Model file for the job. Use its own axes, mm. Face numbers are marked on the shaded views. A direction names the side the tool comes from. Coordinates: 2 decimals unless noted, no trailing zeros. Write each loop counter-clockwise with the first axis right and the second up, starting at its lowest first coordinate (ties: lowest second). Pieces come first, ordered by that corner, then holes.
Q1. Drill centre lines: probe 1 along X at (y, z) = (12.25, 13); probe 2 along Y at (x, z) = (9.75, 16.75); probe 3 along Z at (x, y) = (12.5, 19.5). Where is each one in solid material? Low to high.
Q2. Which spindle directions (+Z, -Z, +X, -X, +Y, -Y) get a long thin tool onto all of the face, cutting with end or side? Do the marked faces 5, 6, 7, 8 and 9. Say none if no direction does.
Q3. Band-saw the part on C-C, the plane z = 17.5. Write the cut outline in (x, y).
Q4. Pull direction Y, two halves, no side cores. Call the marked faces 1, 2, 3 and 4: released by +Y, released by -Y, zero draft, split by the parting line, or undercut.
Q5. Band-saw the part on B-B, the plane y = 10.5. Write the cut outline in (x, z) (3 decimals), plus the area to 3 significant figures.
Q6. Band-saw the part on D-D, the plane y = 2.5. Write the cut outline in (x, z), plus the area to 3 significant figures.
Q7. Band-saw the part on A-A, the plane x = 8.25. Write the cut outline in (y, z).
Q8. Pin check, flat tips, straight feed: P1, Ø3.5, axis at x = 9, y = 16.5, coming from the -Z side; P2, Ø3.5, axis at x = 7.5, z = 8.5, coming from the +Y side. Stop position of each tip, or through.
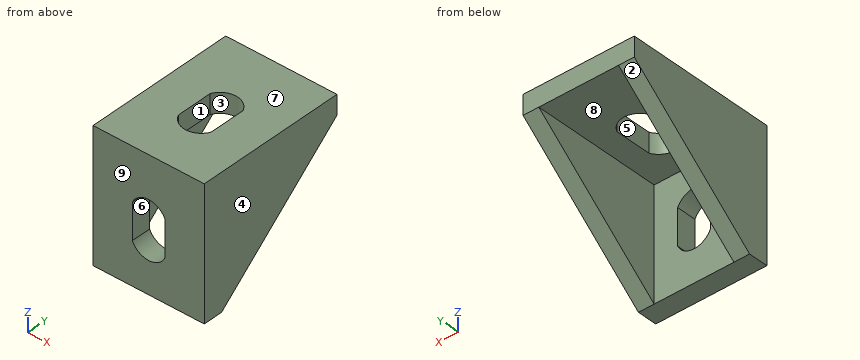
Autodesk Inventor part; units mm, degrees
ref_plane "YZ Plane" through (0, 0, 0) normal (1, 0, 0) x (0, 1, 0)
ref_plane "XZ Plane" through (0, 0, 0) normal (0, 1, 0) x (-1, 0, 0)
ref_plane "XY Plane" through (0, 0, 0) normal (0, 0, 1) x (1, 0, 0)
sketch "Sketch1" plane through (0, 0, 0) normal (0, 0, 1) x (1, 0, 0)
  line L0 (0, 0) -> (0, 3)
  line L1 (0, 3) -> (17, 3)
  line L2 (17, 3) -> (17, 0)
  line L3 (17, 0) -> (0, 0)
  dimension "d0" = 3
  dimension "d1" = 17
extrude "Extrusion1" add sketch "Sketch1" along normal blind 20
sketch "Sketch2" plane through (17, 0, 0) normal (1, 0, 0) x (0, 0, -1)
  point P0 (0, 0)
sketch "Sketch3" plane through (0, 3, 0) normal (0, 1, 0) x (1, 0, 0)
  line L0 (17, -20) -> (17, -17)
  line L1 (17, 0) -> (17, -20)
  line L2 (17, -17) -> (0, -17)
  line L3 (0, 0) -> (0, -20)
  line L4 (17, -20) -> (0, -20)
  line L5 (0, -20) -> (0, -17)
  line L6 (0, -20) -> (17, -20)
  dimension "d4" = 3
extrude "Extrusion2" add sketch "Sketch3" along normal blind 20
sketch "Sketch4" plane through (17, 0, 0) normal (1, 0, 0) x (0, 0, -1)
  line L0 (-20, 23) -> (-17, 23)
  line L1 (0, 3) -> (-17, 23)
  line L2 (0, 3) -> (-17, 3)
  line L3 (-17, 23) -> (-17, 3)
  line L4 (-17, 3) -> (0, 3)
  point P0 (0, 0)
extrude "Extrusion3" add sketch "Sketch4" against normal blind 2.4
sketch "Sketch5" plane through (0, 0, 0) normal (-1, 0, 0) x (0, 0, 1)
  line L0 (17, 3) -> (17, 23)
  line L1 (0, 3) -> (0, 0)
  line L2 (17, 23) -> (0, 3)
  line L3 (0, 3) -> (17, 3)
  line L4 (17, 23) -> (0, 3)
  line L5 (17, 3) -> (17, 23)
extrude "Extrusion4" add sketch "Sketch5" against normal blind 2.4
sketch "Sketch6" plane through (14.6, 3, 17) normal (0, 0, -1) x (-1, 0, 0)
  line L0 (-2.4, -3) -> (-2.4, 20)
  line L1 (-2.4, -3) -> (6.1, -3)
  line L2 (14.6, -3) -> (-2.4, -3)
  line L3 (6.1, 5) -> (6.7519, 5)
  line L4 (6.7519, 10.5) -> (6.1, 10.5)
  line L5 (6.1, 10.5) -> (3.6, 10.5)
  line L6 (3.6, 10.5) -> (8.6, 10.5)
  line L7 (6.1, 5) -> (3.6, 5)
  line L8 (3.6, 5) -> (8.6, 5)
  line L9 (8.6, 5) -> (8.6, 10.5)
  line L10 (3.6, 10.5) -> (3.6, 5)
  arc A0 (8.6, 10.5) -> (3.6, 10.5) centre (6.1, 9.3544) ccw
  arc A1 (3.6, 5) -> (8.6, 5) centre (6.1, 6.1456) ccw
  dimension "d11" = 8.5
extrude "Extrusion5" cut sketch "Sketch6" against normal through all
sketch "Sketch7" plane through (2.4, 3, 17) normal (0, 1, 0) x (1, 0, 0)
  line L0 (-2.4, -3) -> (-2.4, 20)
  line L1 (-2.4, -3) -> (6.1, -3)
  line L2 (14.6, -3) -> (-2.4, -3)
  line L3 (6.1, 5) -> (6.7519, 5)
  line L4 (6.7519, 10.5) -> (6.1, 10.5)
  line L5 (6.1, 10.5) -> (3.6, 10.5)
  line L6 (3.6, 10.5) -> (8.6, 10.5)
  line L7 (6.1, 5) -> (3.6, 5)
  line L8 (3.6, 5) -> (8.6, 5)
  line L9 (8.6, 5) -> (8.6, 10.5)
  line L10 (3.6, 10.5) -> (3.6, 5)
  arc A0 (8.6, 10.5) -> (3.6, 10.5) centre (6.1, 9.3544) ccw
  arc A1 (3.6, 5) -> (8.6, 5) centre (6.1, 6.1456) ccw
  dimension "d25" = 8.5
extrude "Extrusion6" cut sketch "Sketch7" against normal through all
properties part number "90 Degree attachment T Slot"
Answer sheet:
1. probe 1: x = 0 to 2.4, 14.6 to 17
1. probe 2: y = 0 to 3
1. probe 3: z = 17 to 20
2. face 5: +Z, -Z
2. face 6: +Y, -Y
2. face 7: +Z, +X, -X, +Y, -Y
2. face 8: -Z, +Y
2. face 9: +Z, -Z, +X, -X, -Y
3. outline: (0, 0) - (17, 0) - (17, 23) - (0, 23) - close; hole (6, 8) arc R2.75 ccw to (11, 8) - (11, 13.5) arc R2.75 ccw to (6, 13.5) - close
4. face 1: undercut
4. face 2: released by +Y
4. face 3: undercut
4. face 4: zero draft
5. outline: (0, 6.375) - (2.4, 6.375) - (2.4, 17) - (6, 17) - (6, 20) - (0, 20) - close; (11, 17) - (14.6, 17) - (14.6, 6.375) - (17, 6.375) - (17, 20) - (11, 20) - close
5. area: 87.0 mm2
6. outline: (0, 0) - (17, 0) - (17, 20) - (0, 20) - close; hole (6, 6.5) arc R2.75 ccw to (11, 6.5) - (11, 12) arc R2.75 ccw to (6, 12) - close
6. area: 301 mm2
7. outline: (0, 0) - (3, 0) - (3, 4.91) - (0, 4.91) - close; (0, 13.59) - (3, 13.59) - (3, 17) - (6.41, 17) - (6.41, 20) - (0, 20) - close; (15.09, 17) - (23, 17) - (23, 20) - (15.09, 20) - close
8. P1: stops at z = 17
8. P2: stops at y = 3
